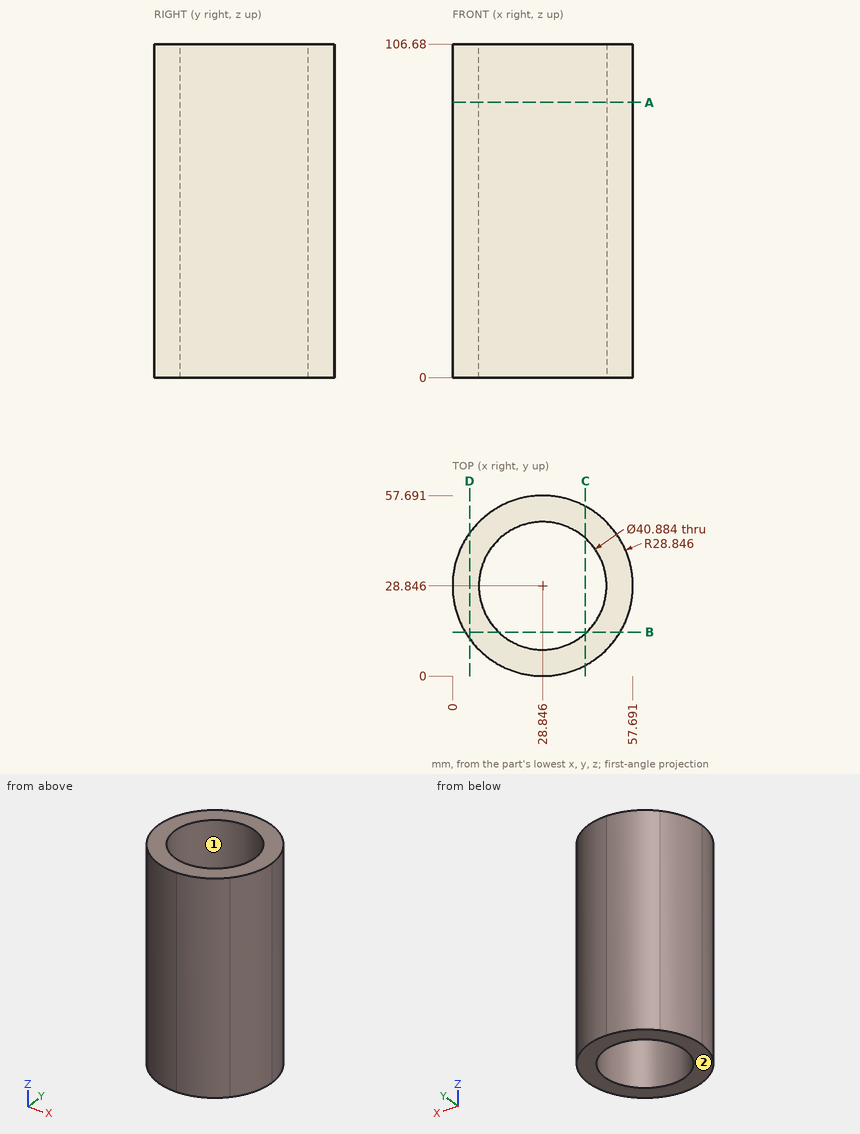
Here's the drawing with two shaded views (mm, measured from the low corner). I have some questions. Coordinates: 2 decimals unless noted, no trailing zeros. Order: outer loops, then holes, each group sorted by start corner. A loop starts at its lowest first (then second) coordinate and runs counter-clockwise, first axis right, second up.
Q1. Suppose I cut it at D-D on x = 5.5. Please give me the cut outline in (y, z).
Q2. Suppose I cut it at C-C on x = 42.5. Please give me the cut outline in (y, z) (1 decimal), and give its area (3 significant figures).
Q3. Suppose I cut it at B-B on y = 14. Please give me the cut outline in (x, z), and give its area (3 significant figures).
Q4. Thinking about a two-plate mould opening in X: for the marked faces 1 and 2, which applies, released by +X, released by -X, zero draft, split by the parting line, or undercut?
Q5. Will these pins go through, and if not, where does the flat tip stop? pin 1 (4 mm diameter, centred on y = 48.5, z = 25, fed in from +X); pin 2 (10 mm diameter, centred on x = 14, z = 63, fed in from +Y); pin 3 (6 mm diameter, centred on y = 24, z = 71.5, fed in from +X).
Q6. Please list where these lines run through material, in increasing order: L1, parallel to X at y = 19.5, z = 100 (1 decimal); L2, parallel to Y at x = 28, z = 35.5; L3, parallel to Y at x = 17, z = 26 (1 decimal).
Q7. Suppose I cut it at A-A on z = 88. Please give me the cut outline in (x, y) (1 decimal), and give its area (3 significant figures).
Answer:
1. outline: (11.9, 0) - (45.79, 0) - (45.79, 106.68) - (11.9, 106.68) - close
2. outline: (3.4, 0) - (13.6, 0) - (13.6, 106.7) - (3.4, 106.7) - close; (44.1, 0) - (54.3, 0) - (54.3, 106.7) - (44.1, 106.7) - close
2. area: 2,180 mm2
3. outline: (4.11, 0) - (14.79, 0) - (14.79, 106.68) - (4.11, 106.68) - close; (42.9, 0) - (53.58, 0) - (53.58, 106.68) - (42.9, 106.68) - close
3. area: 2,280 mm2
4. face 1: undercut
4. face 2: zero draft
5. pin 1: stops at x = 51.66
5. pin 2: stops at y = 55.96
5. pin 3: stops at x = 57.63
6. L1: x = 1.6 to 10.7, 47 to 56.1
6. L2: y = 0.01 to 8.42, 49.27 to 57.68
6. L3: y = 2.5 to 12.2, 45.5 to 55.1
7. outline: (0, 28.8) arc R28.8 ccw to (9, 7.9) arc R28.8 ccw to (28.8, 0) arc R28.8 ccw to (49.8, 9) arc R28.8 ccw to (57.7, 28.8) arc R28.8 ccw to (48.7, 49.8) arc R28.8 ccw to (28.8, 57.7) arc R28.8 ccw to (7.9, 48.7) arc R28.8 ccw to start; hole circle Ø40.9 at (28.8, 28.8)
7. area: 1,300 mm2
